```python
from build123d import *

# Parameters (mm, degrees)
PAD003_DEPTH    = 10
SKETCH008_W     = 13.2
SKETCH008_H     = 1.8
POCKET005_DEPTH = 10
SKETCH011_R     = 5.1
PAD005_DEPTH    = 2
SKETCH012_R     = 4.35
POCKET006_DEPTH = 6
SKETCH013_W     = 15.4
SKETCH013_H     = 4.4
PAD006_DEPTH    = 0.6


with BuildPart() as part:
    # Sketch006 → Revolution (revolve)
    with BuildSketch(Plane.YZ):
        Polygon((-4, 26.637276), (-12, 20), (-12, 0), (-13.6, 0), (-13.6, 21.046803), (-4, 28.637276), (0, 28.637276), (0, 26.637276), align=None)
    revolve(axis=Axis((0, 0, 0), (0, 0, 1)))

    # Sketch007 (on Face3 of Revolution) → Pad003 (new body)
    with BuildSketch(Plane.YX):
        Polygon((-12.6, 2.2), (1.2, 2.2), (1.2, 12.3), (2.8, 12.3), (2.8, -12.3), (1.2, -12.3), (1.2, -2.2), (-12.6, -2.2), align=None)
    extrude(amount=-PAD003_DEPTH)

    # Sketch008 → Pocket005 (cut)
    with BuildSketch(Plane.YX):
        with Locations((-5.2, 0)):
            Rectangle(SKETCH008_W, SKETCH008_H)
    extrude(amount=-POCKET005_DEPTH, mode=Mode.SUBTRACT)

    # Sketch011 → Pad005 (join, symmetric)
    with BuildSketch(Plane(origin=(0, 0, 28.637276), x_dir=(0, -1, 0), z_dir=(0, 0, 1))):
        Circle(SKETCH011_R)
    extrude(amount=PAD005_DEPTH, both=True)

    # Sketch012 (on Face22 of Pad005) → Pocket006 (cut)
    with BuildSketch(Plane(origin=(0, 0, 30.637276), x_dir=(0, -1, 0), z_dir=(0, 0, 1))):
        Circle(SKETCH012_R)
    extrude(amount=-POCKET006_DEPTH, mode=Mode.SUBTRACT)

    # Sketch013 (on Face5 of Pocket006) → Pad006 (join)
    with BuildSketch(Plane(origin=(0, 0, 10), x_dir=(0, -1, 0), z_dir=(0, 0, 1))):
        with Locations((5.497757, 0)):
            Rectangle(SKETCH013_W, SKETCH013_H)
    extrude(amount=PAD006_DEPTH)


solid = part.part
```
The model under review builds one solid part; all positions refer to its coordinate system, in mm. A direction names the side the tool comes from. Round coordinates to 2 decimals unless told otherwise and drop trailing zeros. Write each loop counter-clockwise with the first axis right and the second up, starting at its lowest first coordinate (ties: lowest second). Pieces come first, ordered by that corner, then holes. Notation, with made-up numbers: (-6.75, 30) - (-1.75, 30) arc R18 cw to (-1.75, 50) - close; hole circle Ø10 at (-22.75, 68.25). An arc over 180 degrees is marked (long way). Answer as CSV lines item,"result". Start each with the question number.
(1) For faces 4 (the flat face through (-7, 1.2, 5)), 5 (the cylindrical face through (-4.247, 0.943, 28.522)), 6 (the conical face through (-4.71, 1.05, 25.95)), list the 3-axis set-ups (+Z, -Z, +X, -X, +Y, -Y) from which the entire face can be reached by the end or side of a thin tool; tool diameter is ignored.
(2) We need section D-D on z = 14.5. State the section outline as (x, y) points, plus the area to 3 significant figures.
(3) We need section C-C on x = 0. State the section outline as (y, z) points, plus the area to 3 significant figures.
(4) Draft analysis for pull direction Y (two halves, no side actions). For faces 1 (the cylindrical face through (-4.5, -2.4, 29.2)), 2 (the flat face through (-0.9, -5, 5)), 3 (the flat face through (-2, 0, 0)), state which applies: pulls with the +Y half, pulls with the -Y half, needs draft (parallel to the pull), parting line crosses it, or undercut.
(5) We need section B-B on z = 7. State the section outline as (x, y) points, plus the area to 3 significant figures.
(6) We need section A-A on y = 0. State the section outline as (x, z) points, plus the area to 3 significant figures.
(7) To check wall thickness, follow line 1 (Y direction, x = -0.25, z = 4.5); line 2 (X direction, y = 0, z = 11). State the ranges of each line that lie inside material, in increasing order.
(8) For pin 1 Ø2 at (x, z) = (-9.5, 8) entering from -Y; pin 2 Ø5 at (x, z) = (-5, 15) entering from -Y; pin 3 Ø5 at (y, z) = (-7, 4.5) entering from +X, all flat-tipped, find the tip position at first contact; note any pin that passes through.
Worked answers:
1,face 4,"-Z"
1,face 5,"+Z"
1,face 6,"none"
2,outline,"circle Ø27.2 at (0, 0); hole circle Ø24 at (0, 0)"
2,area,"129 mm²"
3,outline,"(-13.6, 0) - (-11.8, 0) - (-11.8, 10) - (1.4, 10) - (1.4, 0) - (2.8, 0) - (2.8, 10) - (2.2, 10) - (2.2, 10.6) - (-12, 10.6) - (-12, 20) - (-4.35, 26.35) - (-4.35, 30.64) - (-5.1, 30.64) - (-5.1, 27.77) - (-13.6, 21.05) - close; (4.35, 26.35) - (12, 20) - (12, 0) - (13.6, 0) - (13.6, 21.05) - (5.1, 27.77) - (5.1, 30.64) - (4.35, 30.64) - close"
3,area,"131 mm²"
4,face 1,"parting line crosses it"
4,face 2,"undercut"
4,face 3,"needs draft"
5,outline,"circle Ø27.2 at (0, 0); hole (-11.94, 1.2) arc R12 ccw to (-2.2, -11.8) - (-2.2, 1.2) - close; hole (-11.67, 2.8) - (11.67, 2.8) arc R12 ccw to start; hole (-0.9, -11.8) - (0.9, -11.8) - (0.9, 1.4) - (-0.9, 1.4) - close; hole (2.2, -11.8) arc R12 ccw to (11.94, 1.2) - (2.2, 1.2) - close"
5,area,"201 mm²"
6,outline,"(-13.6, 0) - (-12, 0) - (-12, 20) - (-4.35, 26.35) - (-4.35, 30.64) - (-5.1, 30.64) - (-5.1, 27.77) - (-13.6, 21.05) - close; (-2.2, 0) - (-0.9, 0) - (-0.9, 10) - (0.9, 10) - (0.9, 0) - (2.2, 0) - (2.2, 10.6) - (-2.2, 10.6) - close; (4.35, 26.35) - (12, 20) - (12, 0) - (13.6, 0) - (13.6, 21.05) - (5.1, 27.77) - (5.1, 30.64) - (4.35, 30.64) - close"
6,area,"135 mm²"
7,line 1,"-13.6 to -11.8, 1.4 to 2.8, 12 to 13.6"
7,line 2,"-13.6 to -12, 12 to 13.6"
8,pin 1,"y = -10.62"
8,pin 2,"y = -13.37"
8,pin 3,"x = 12.83"
